The listing builds one solid part. Answer for the finished solid, in the listing's coordinates (mm). A direction names the side the tool comes from. Coordinates: 2 decimals unless noted, no trailing zeros. Write each loop counter-clockwise with the first axis right and the second up, starting at its lowest first coordinate (ties: lowest second). Pieces come first, ordered by that corner, then holes.
(1) Which of the six approach directions +Z, -Z, +X, -X, +Y, -Y give full straight-line access (tool end or side, diameter ignored) to faces 1 (the flat face through (414.726, 305.21, -351.982)), 2 (the flat face through (582, 500, -7)), 3 (the flat face through (-539.554, 305.21, -355.949))?
(2) The part is cut by section B-B on z = 283. Determine the outline of the cut face in (x, y), plus the area to 3 significant figures.
(3) Straight lines are drawn through the part: line 1 (Y direction, x = -101.5, z = -209.5); line 2 (X direction, y = 299.5, z = -287); line 3 (X direction, y = 408, z = -127.5). For each, find the intervals that lie inside material, in ascending order.
(4) The part is cut by section D-D on z = 17. Determine the outline of the cut face in (x, y).
(5) The part is cut by section A-A on y = 385. Determine the outline of the cut face in (x, z), plus the area to 3 significant figures.
(6) The part is cut by section C-C on x = 457.5. Determine the outline of the cut face in (y, z).
(7) For a pull along Z with two mould halves and no side action, classify faces 4 (the flat face through (732, 305, 352)), 5 (the flat face through (-530, 290, 356)), 6 (the flat face through (530, 270, -310.5)) as +Z half, -Z half, draft (parallel to the pull), parting line (faces both ways), or undercut.
from build123d import *

# Parameters (mm, degrees)
SKETCH_1_W               = 2060
SKETCH_1_H               = 800
EXTRUDE_1_DEPTH          = 500
SKETCH_3_W               = 220
SKETCH_3_H               = 220
CUT_EXTRUDE_1_DEPTH      = 310.5
EXTRUDE_2_REACH          = 2159.22
SKETCH_5_W               = 220
SKETCH_5_H               = 210
CUT_EXTRUDE_2_DEPTH      = 1399.18310675
SKETCH_7_W               = 220
SKETCH_7_H               = 210
CUT_EXTRUDE_3_DEPTH      = 1330.488578602
CUT_EXTRUDE_3_DEPTH_BACK = 1330.488578602
CUT_EXTRUDE_4_DEPTH      = 40
SKETCH_14_W              = 220
SKETCH_14_H              = 210
CUT_EXTRUDE_5_DEPTH      = 1330.488578602
CUT_EXTRUDE_5_DEPTH_BACK = 1330.488578602
CUT_EXTRUDE_6_DEPTH      = 40
SKETCH_16_W              = 35.606145385
SKETCH_16_H              = 210
CUT_EXTRUDE_7_DEPTH      = 1399.18310675
CUT_EXTRUDE_7_DEPTH_BACK = 1399.18310675
SKETCH_18_W              = 35.606145385
SKETCH_18_H              = 210
CUT_EXTRUDE_11_DEPTH     = 1399.18310675
CUT_EXTRUDE_12_DEPTH     = 40
CUT_EXTRUDE_15_DEPTH     = 2159.151060515
CHAMFER_1_SIZE           = 30
CUT_EXTRUDE_16_DEPTH     = 40
CHAMFER_2_SIZE           = 30


with BuildPart() as part:
    # 草图1 → 凸台-拉伸1 (new body)
    with BuildSketch(Plane(origin=(0, 0, 0), x_dir=(1, 0, 0), z_dir=(0, 1, 0))):
        Rectangle(SKETCH_1_W, SKETCH_1_H)
    extrude(amount=EXTRUDE_1_DEPTH)

    # 草图3 → 切除-拉伸1 (cut, symmetric)
    with BuildSketch(Plane.XY):
        with Locations((0, 360)):
            Rectangle(SKETCH_3_W, SKETCH_3_H)
    extrude(amount=CUT_EXTRUDE_1_DEPTH, both=True, mode=Mode.SUBTRACT)

    # 凸台-拉伸2: up to this face of the body (flat: up to its plane)
    extrude_2_end = Plane(part.part.faces().sort_by_distance((-1030, 250, 0))[0])
    # 草图22 → 凸台-拉伸2 (add, up to the picked face)
    with BuildSketch(Plane(origin=(1030, 0, 0), x_dir=(0, 0, -1), z_dir=(1, 0, 0)), mode=Mode.PRIVATE) as extrude_2_sk1:
        Polygon((-330.467185006, 504), (-400, 290), (400, 290), (330.467185006, 504), align=None)
    extrude_2_tool1 = split(extrude(extrude_2_sk1.sketch, amount=-EXTRUDE_2_REACH, mode=Mode.PRIVATE), bisect_by=extrude_2_end, keep=Keep.BOTH, mode=Mode.PRIVATE)
    add(extrude_2_tool1.solids().sort_by(Axis((1030, 393.604907, 0), (-1, 0, 0)))[0])

    # 草图5 → 切除-拉伸2 (cut, through all)
    with BuildSketch(Plane.XY.offset(400)):
        with Locations((0, 395)):
            Rectangle(SKETCH_5_W, SKETCH_5_H)
    extrude(amount=-CUT_EXTRUDE_2_DEPTH, mode=Mode.SUBTRACT)

    # 草图7 → 切除-拉伸3 (cut, two sides)
    with BuildSketch(Plane(origin=(37.34572837, 0, 211.798150344), x_dir=(0.9848077530122092, 0, -0.1736481776669237), z_dir=(0.1736481776669237, 0, 0.9848077530122092))) as cut_extrude_3_sk:
        with Locations((-564.756921873, 395)):
            Rectangle(SKETCH_7_W, SKETCH_7_H)
    extrude(amount=CUT_EXTRUDE_3_DEPTH, mode=Mode.SUBTRACT)
    extrude(cut_extrude_3_sk.sketch, amount=-CUT_EXTRUDE_3_DEPTH_BACK, mode=Mode.SUBTRACT)

    # 草图10 → 切除-拉伸4 (cut)
    with BuildSketch(Plane(origin=(0, 290, 0), x_dir=(1, 0, 0), z_dir=(0, 1, 0))):
        Polygon((-614.635342741, -310.5), (-407.022752899, -310.5), (-516.521807919, 310.5), (-739.915662534, 310.5), (-630.416607514, -310.5), align=None)
    extrude(amount=-CUT_EXTRUDE_4_DEPTH, mode=Mode.SUBTRACT)

    # 草图14 → 切除-拉伸5 (cut, two sides)
    with BuildSketch(Plane(origin=(37.34572837, 0, 211.798150344), x_dir=(0.9848077530122092, 0, -0.1736481776669237), z_dir=(0.1736481776669237, 0, 0.9848077530122092))) as cut_extrude_5_sk:
        with Locations((564.756921873, 395)):
            Rectangle(SKETCH_14_W, SKETCH_14_H)
    extrude(amount=CUT_EXTRUDE_5_DEPTH, mode=Mode.SUBTRACT)
    extrude(cut_extrude_5_sk.sketch, amount=-CUT_EXTRUDE_5_DEPTH_BACK, mode=Mode.SUBTRACT)

    # 草图15 → 切除-拉伸6 (cut)
    with BuildSketch(Plane(origin=(0, 290, 0), x_dir=(1, 0, 0), z_dir=(0, 1, 0))):
        Polygon((630.416607514, 310.5), (407.022752899, 310.5), (516.521807919, -310.5), (739.915662534, -310.5), align=None)
    extrude(amount=-CUT_EXTRUDE_6_DEPTH, mode=Mode.SUBTRACT)

    # 草图16 → 切除-拉伸7 (cut, two sides)
    with BuildSketch(Plane(origin=(0, 0, -400), x_dir=(-1, 0, 0), z_dir=(0, 0, -1))) as cut_extrude_7_sk:
        with Locations((-632.438415434, 395)):
            Rectangle(SKETCH_16_W, SKETCH_16_H)
    extrude(amount=CUT_EXTRUDE_7_DEPTH, mode=Mode.SUBTRACT)
    extrude(cut_extrude_7_sk.sketch, amount=-CUT_EXTRUDE_7_DEPTH_BACK, mode=Mode.SUBTRACT)

    # 草图18 → 切除-拉伸11 (cut, through all)
    with BuildSketch(Plane.XY.offset(400)):
        with Locations((-632.438415434, 395)):
            Rectangle(SKETCH_18_W, SKETCH_18_H)
    extrude(amount=-CUT_EXTRUDE_11_DEPTH, mode=Mode.SUBTRACT)

    # 草图19 → 切除-拉伸12 (cut)
    with BuildSketch(Plane(origin=(0, 290, 0), x_dir=(1, 0, 0), z_dir=(0, 1, 0))):
        Polygon((-650.241488126, -310.5), (-630.416607514, -310.5), (-650.241488126, -198.067515011), align=None)
    extrude(amount=-CUT_EXTRUDE_12_DEPTH, mode=Mode.SUBTRACT)

    # 草图23 → 切除-拉伸15 (cut, through all)
    with BuildSketch(Plane(origin=(1030, 0, 0), x_dir=(0, 0, -1), z_dir=(1, 0, 0))):
        Polygon((400, 500), (400, 290), (331.766863791, 500), align=None)
        Polygon((-400, 500), (-400, 290), (-331.766863791, 500), align=None)
    extrude(amount=-CUT_EXTRUDE_15_DEPTH, mode=Mode.SUBTRACT)

    # 倒角1
    chamfer_1_edges = [part.edges().sort_by_distance(p)[0] for p in [
        (-399.132120513, 290, 355.25),
        (524.412440306, 290, 355.25),
        (747.806294921, 290, 355.25),
        (-650.241488126, 290, 355.25),
        (110, 290, 355.25),
        (-110, 290, 355.25),
    ]]
    chamfer(chamfer_1_edges, length=CHAMFER_1_SIZE)

    # 草图24 → 切除-拉伸16 (cut)
    with BuildSketch(Plane(origin=(0, 290, 0), x_dir=(1, 0, 0), z_dir=(0, 1, 0))):
        Polygon((650.241488126, 310.5), (630.416607514, 310.5), (650.241488126, 198.067515011), align=None)
    extrude(amount=-CUT_EXTRUDE_16_DEPTH, mode=Mode.SUBTRACT)

    # 倒角2
    chamfer_2_edges = [part.edges().sort_by_distance(p)[0] for p in [
        (399.132120513, 290, -355.25),
        (650.241488126, 290, -355.25),
        (110, 290, -355.25),
        (-110, 290, -355.25),
        (-524.412440306, 290, -355.25),
        (-747.806294921, 290, -355.25),
    ]]
    chamfer(chamfer_2_edges, length=CHAMFER_2_SIZE)


solid = part.part
Model answer:
1. face 1: -Z
1. face 2: none
1. face 3: +Z
2. outline: (-1030, 0) - (1030, 0) - (1030, 504) - (-1030, 504) - close; hole (-650.24, 250) - (-411.87, 250) - (-411.87, 500) - (-650.24, 500) - close; hole (-110, 250) - (110, 250) - (110, 500) - (-110, 500) - close; hole (511.67, 250) - (735.07, 250) - (735.07, 500) - (511.67, 500) - close
2. area: 868,000 mm2
3. line 1: y = 0 to 250, 500 to 504
3. line 2: x = -1030 to -735.77, -512.38 to -110, 110 to 411.17, 650.24 to 1030
3. line 3: x = -1030 to -707.65, -484.25 to -110, 110 to 439.29, 662.68 to 1030
4. outline: (-1030, 0) - (1030, 0) - (1030, 504) - (-1030, 504) - close; hole (-682.17, 250) - (-458.77, 250) - (-458.77, 500) - (-682.17, 500) - close; hole (-110, 250) - (110, 250) - (110, 500) - (-110, 500) - close; hole (464.77, 250) - (688.16, 250) - (688.16, 500) - (464.77, 500) - close
5. outline: (-1030, -369.13) - (-750.25, -369.13) - (-650.24, 198.07) - (-650.24, 369.13) - (-1030, 369.13) - close; (-526.86, -369.13) - (-110, -369.13) - (-110, 369.13) - (-396.68, 369.13) - close; (110, -369.13) - (396.68, -369.13) - (526.86, 369.13) - (110, 369.13) - close; (650.24, -369.13) - (1030, -369.13) - (1030, 369.13) - (750.25, 369.13) - (650.24, -198.07) - close
5. area: 1,020,000 mm2
6. outline: (0, -400) - (290, -400) - (290, -310.5) - (250, -310.5) - (250, -24.23) - (500, -24.23) - (500, -331.77) - (504, -330.47) - (504, 330.47) - (290, 400) - (0, 400) - close
7. face 4: +Z half
7. face 5: draft
7. face 6: undercut
